Read the model definition and answer for the solid it produces. Units are mm, in the model's axes. Face numbers are marked on the shaded views. A direction names the side the tool comes from. Coordinates: 2 decimals unless noted, no trailing zeros. Loops run counter-clockwise (first coordinate to the right, second up) from the corner with the lowest first, then second, coordinate; pieces in that order, holes last.
from build123d import *

# Parameters (mm, degrees)
SKETCH2_W                 = 70
SKETCH2_H                 = 70
BOSS_EXTRUDE1_DEPTH       = 6.35
CHAMFER1_SIZE             = 10
SKETCH3_R                 = 1.5
CUT_EXTRUDE1_DEPTH        = 13.7
M4_CLEARANCE_HOLE1_D      = 4.5
CUT_EXTRUDE2_DEPTH        = 13.7
FILLET1_R                 = 100
CUT_EXTRUDE3_DEPTH        = 13.7
M4X0_7_TAPPED_HOLE1_D     = 3.3
M4X0_7_TAPPED_HOLE1_DEPTH = 13
M4X0_7_TAPPED_HOLE1_TIP   = 0.991420021
M4X0_7_TAPPED_HOLE2_D     = 3.3
M2X0_4_TAPPED_HOLE1_D     = 1.6
M2X0_4_TAPPED_HOLE1_DEPTH = 12
M2X0_4_TAPPED_HOLE1_TIP   = 0.480688495


with BuildPart() as part:
    # Sketch2 → Boss-Extrude1 (new body, symmetric)
    with BuildSketch(Plane.XY):
        Rectangle(SKETCH2_W, SKETCH2_H)
    extrude(amount=BOSS_EXTRUDE1_DEPTH, both=True)

    # Chamfer1
    chamfer1_edges = [part.edges().sort_by_distance(p)[0] for p in [
        (-35, 35, 0),
        (35, 35, 0),
    ]]
    chamfer(chamfer1_edges, length=CHAMFER1_SIZE)

    # Sketch3 → Cut-Extrude1 (cut, through all)
    with BuildSketch(Plane(origin=(0, 0, -6.35), x_dir=(-1, 0, 0), z_dir=(0, 0, -1))):
        with Locations((0, 5)):
            Circle(SKETCH3_R)
    extrude(amount=-CUT_EXTRUDE1_DEPTH, mode=Mode.SUBTRACT)

    # M4 Clearance Hole1 (through all)
    with Locations(Plane(origin=(0, 0, -6.35), x_dir=(-1, 0, 0), z_dir=(0, 0, -1))):
        with Locations((5.75, 14.959292144), (-5.75, 14.959292144), (-11.5, 5), (-5.75, -4.959292144), (5.75, -4.959292144), (11.5, 5)):
            Hole(M4_CLEARANCE_HOLE1_D / 2)

    # Sketch6 → Cut-Extrude2 (cut, through all)
    with BuildSketch(Plane(origin=(0, 0, -6.35), x_dir=(-1, 0, 0), z_dir=(0, 0, -1))):
        with BuildLine():
            Line((-35, -27.5), (-22.5, 5))
            ThreePointArc((-22.5, 5), (0, 27.5), (22.5, 5))
            Line((22.5, 5), (35, -27.5))
            Line((35, -27.5), (35, 25))
            Line((35, 25), (25, 35))
            Line((25, 35), (-25, 35))
            Line((-25, 35), (-35, 25))
            Line((-35, 25), (-35, -27.5))
        make_face()
    extrude(amount=-CUT_EXTRUDE2_DEPTH, mode=Mode.SUBTRACT)

    # Fillet1
    fillet1_edges = [part.edges().sort_by_distance(p)[0] for p in [
        (-22.5, 5, 0),
        (22.5, 5, 0),
    ]]
    fillet(fillet1_edges, radius=FILLET1_R)

    # Sketch7 → Cut-Extrude3 (cut, through all)
    with BuildSketch(Plane(origin=(0, 0, -6.35), x_dir=(-1, 0, 0), z_dir=(0, 0, -1))):
        with BuildLine():
            Line((-10, -35), (10, -35))
            Line((10, -35), (10, -33))
            ThreePointArc((10, -33), (7.656854249, -27.343145751), (2, -25))
            Line((2, -25), (-2, -25))
            ThreePointArc((-2, -25), (-7.656854249, -27.343145751), (-10, -33))
            Line((-10, -33), (-10, -35))
        make_face()
    extrude(amount=-CUT_EXTRUDE3_DEPTH, mode=Mode.SUBTRACT)

    # M4x0.7 Tapped Hole1
    with Locations(Plane(origin=(0, -35, 0), x_dir=(-1, 0, 0), z_dir=(0, -1, 0))):
        with Locations((-27.5, 0), (-17.5, 0), (17.5, 0), (27.5, 0)):
            Hole(M4X0_7_TAPPED_HOLE1_D / 2, depth=M4X0_7_TAPPED_HOLE1_DEPTH)
            with Locations((0, 0, -(M4X0_7_TAPPED_HOLE1_DEPTH + M4X0_7_TAPPED_HOLE1_TIP / 2))):  # 118° drill point
                Cone(0, M4X0_7_TAPPED_HOLE1_D / 2, M4X0_7_TAPPED_HOLE1_TIP, mode=Mode.SUBTRACT)

    # M4x0.7 Tapped Hole2 (through all)
    with Locations(Plane(origin=(0, 0, -6.35), x_dir=(-1, 0, 0), z_dir=(0, 0, -1))):
        with Locations((12.662387957, -23.625), (22.662387957, -23.625)):
            Hole(M4X0_7_TAPPED_HOLE2_D / 2)

    # M2x0.4 Tapped Hole1
    with Locations(Plane(origin=(35, 0, 0), x_dir=(0, 0, -1), z_dir=(1, 0, 0))):
        with Locations((-4.765, -28.5), (4.765, -28.5)):
            Hole(M2X0_4_TAPPED_HOLE1_D / 2, depth=M2X0_4_TAPPED_HOLE1_DEPTH)
            with Locations((0, 0, -(M2X0_4_TAPPED_HOLE1_DEPTH + M2X0_4_TAPPED_HOLE1_TIP / 2))):  # 118° drill point
                Cone(0, M2X0_4_TAPPED_HOLE1_D / 2, M2X0_4_TAPPED_HOLE1_TIP, mode=Mode.SUBTRACT)


solid = part.part
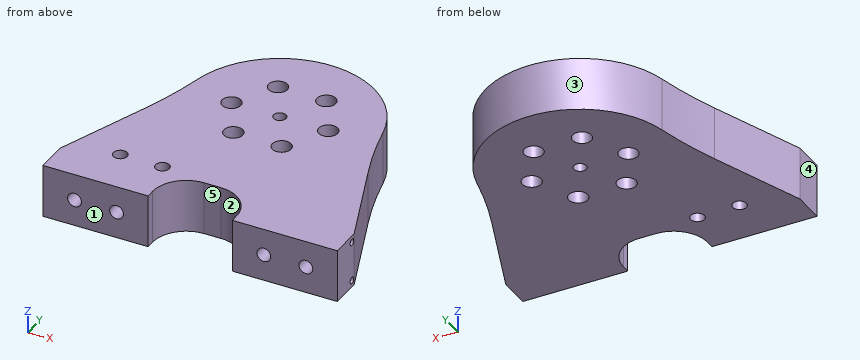
Item 1: Given pin 1 (2 mm diameter, centred on x = -27.5, z = 0, fed in from -Y); pin 2 (2.5 mm diameter, centred on x = 0, y = 5, fed in from -Z); pin 3 (5 mm diameter, centred on x = -5, z = 2, fed in from +Y); pin 4 (1.2 mm diameter, centred on x = 0, z = 0.5, fed in from -Y), each flat-ended and moving along its own axis, determine where each tip first touches the part or whether it passes through.
Numbers:
pin 1: stops at y = -21.61
pin 2: passes through
pin 3: stops at y = 27.36
pin 4: stops at y = -25
Item 2: Determine the mould class of the marked faces 3, 4 and 5 for opening direction X: released by +X, released by -X, zero draft, split by the parting line, or undercut.
Numbers:
face 3: split by the parting line
face 4: released by -X
face 5: undercut
Item 3: A cutting plane is placed at A-A on x = 0. Determine the outline of the cut face in (y, z).
Numbers:
outline: (-25, -6.35) - (3.5, -6.35) - (3.5, 6.35) - (-25, 6.35) - close; (6.5, -6.35) - (27.5, -6.35) - (27.5, 6.35) - (6.5, 6.35) - close
Item 4: A cutting plane is placed at B-B on y = 5. Determine the outline of the cut face in (x, z).
Numbers:
outline: (-23.13, -6.35) - (-13.75, -6.35) - (-13.75, 6.35) - (-23.13, 6.35) - close; (-9.25, -6.35) - (-1.5, -6.35) - (-1.5, 6.35) - (-9.25, 6.35) - close; (1.5, -6.35) - (9.25, -6.35) - (9.25, 6.35) - (1.5, 6.35) - close; (13.75, -6.35) - (23.13, -6.35) - (23.13, 6.35) - (13.75, 6.35) - close
Item 5: A cutting plane is placed at D-D on x = 11.5. Determine the outline of the cut face in (y, z).
Numbers:
outline: (-35, -6.35) - (2.75, -6.35) - (2.75, 6.35) - (-35, 6.35) - close; (7.25, -6.35) - (24.34, -6.35) - (24.34, 6.35) - (7.25, 6.35) - close
Item 6: A cutting plane is placed at C-C on y = -14.5. Determine the outline of the cut face in (x, z).
Numbers:
outline: (-30, -6.35) - (30, -6.35) - (30, 6.35) - (-30, 6.35) - close
Item 7: Which of the six approach directions +Z, -Z, +X, -X, +Y, -Y give full straight-line access (tool end or side, diameter ignored) to the marked faces 1 and 2?
Numbers:
face 1: +Z, -Z, +X, -X, -Y
face 2: +Z, -Z, -Y
Item 8: Find the intervals of material crossed by line 1 along X through (y, z) = (-23, 5.5); line 2 along X through (y, z) = (-5, -2.75); line 3 along Y through (x, z) = (-5.75, -0.25), in increasing order.
Numbers:
line 1: x = -33.27 to -24.19, -21.14 to -14.19, -11.14 to 33.27
line 2: x = -26.35 to -8, -3.5 to 3.5, 8 to 26.35
line 3: y = -25.93 to -7.21, -2.71 to 12.71, 17.21 to 26.75
